Could you check a few things on this model? Use its own coordinates, in mm. Round coordinates to 2 decimals unless told otherwise and drop trailing zeros. Write each loop counter-clockwise with the first axis right and the second up, starting at its lowest first coordinate (ties: lowest second). Pieces come first, ordered by that corner, then holes. Notation, with made-up numbers: (11.25, 89.25) -> (17.25, 89.25) arc R25 cw to (17.25, 106.25) -> close; hole circle Ø1 at (-18, 24). An arc over 180 degrees is marked (long way). One line per question, with ' | ' between items. Start each with the question number.
1. Imagine slicing it at C-C, the plane y = -2.25. List the corners of the cut face in (x, z) for me.
2. For pin 1 Ø1.5 at (x, z) = (1, 5.5) entering from +Y; pin 2 Ø1 at (x, y) = (-1, 5.5) entering from +Z; pin 3 Ø1.5 at (x, y) = (0.5, 5) entering from -Z, each with a flat end and sliding along its axis, tell me the tip position at first contact or that it passes through.
3. Imagine slicing it at D-D, the plane y = -10.5. List the corners of the cut face in (x, z) for me, and give its area (3 significant figures).
4. Imagine slicing it at B-B, the plane z = -8.25. List the corners of the cut face in (x, y) for me, and give its area (3 significant figures).
5. Imagine slicing it at A-A, the plane x = 1. State how many separate pieces and enclosed holes the cut face has, and give its area (3 significant figures).
6. If I drill on line 1 along Y through (x, z) = (-2.25, 2.5); line 2 along Z through (x, y) = (2.25, 0); line 3 along Y through (x, z) = (1, 8.25), over which ranges is the centre line in solid material (lowest first)? Write a range as [from, to].
Autodesk Inventor part; units mm, degrees
ref_plane "YZ Plane" through (0, 0, 0) normal (1, 0, 0) x (0, 1, 0)
ref_plane "XZ Plane" through (0, 0, 0) normal (0, 1, 0) x (-1, 0, 0)
ref_plane "XY Plane" through (0, 0, 0) normal (0, 0, 1) x (1, 0, 0)
sketch "スケッチ1" plane through (0, 0, 0) normal (1, 0, 0) x (0, 1, 0)
  circle A0 centre (0, 0) radius 14
  dimension "d0" = 28
extrude "押し出し1" add sketch "スケッチ1" along normal mid plane 8
sketch "スケッチ2" plane through (4, 0, 0) normal (1, 0, 0) x (0, 0, -1)
  circle A0 centre (0, 0) radius 14
  circle A1 centre (0, 0) radius 4
  circle A2 centre (0, 0) radius 9
  line L0 (0.25, 3.9922) -> (0.25, 8.9965)
  line L1 (-0.25, 3.9922) -> (-0.25, 8.9965)
  line L2 (2.6461, 2.9997) -> (6.1847, 6.5383)
  line L3 (2.9997, 2.6461) -> (6.5383, 6.1847)
  point P0 (-0.25, 6.4944)
  point P1 (0.25, 6.4944)
  dimension "d3" = 8
  dimension "d4" = 18
  dimension "d5" = 0.5
  dimension "d6" = 0.5
  dimension "d7" = 45
extrude "押し出し2" cut sketch "スケッチ2" against normal through all contours A1 L0 A2 L2
pattern_circular "円形状パターン1" count 8 over 360 about axis through (0, 0, 0) along (1, 0, 0) of "押し出し2"
sketch "スケッチ3" plane through (4, 0, 0) normal (1, 0, 0) x (0, 0, -1)
  circle A0 centre (0, 0) radius 14
hole "穴1" at (4, 0, 0) direction (-1, 0, 0) diameter 2.2 end through all
equation "\"d6\" = d5"
properties part number "wheel"
Geometry results:
1) outline: (-4, -13.82) -> (4, -13.82) -> (4, -8.71) -> (-4, -8.71) -> close; (-4, -3.31) -> (4, -3.31) -> (4, 3.31) -> (-4, 3.31) -> close; (-4, 8.71) -> (4, 8.71) -> (4, 13.82) -> (-4, 13.82) -> close
2) pin 1: stops at y = 13.17 | pin 2: stops at z = 13.08 | pin 3: stops at z = -13.34
3) outline: (-4, -9.26) -> (4, -9.26) -> (4, 9.26) -> (-4, 9.26) -> close | area: 148 mm2
4) outline: (-4, -11.31) -> (4, -11.31) -> (4, -3.6) -> (-4, -3.6) -> close; (-4, -0.25) -> (4, -0.25) -> (4, 0.25) -> (-4, 0.25) -> close; (-4, 3.6) -> (4, 3.6) -> (4, 11.31) -> (-4, 11.31) -> close | area: 127 mm2
5) separate pieces: 1 | enclosed holes: 9 | area: 428 mm2
6) line 1: y = [-13.77, -8.65], [-3.12, 3.12], [8.65, 13.77] | line 2: z = [-14, -1.1], [1.1, 14] | line 3: y = [-11.31, -3.6], [-0.25, 0.25], [3.6, 11.31]
